Answer from the drawing. Dimensions are ordinates in mm from the lowest x, y and z of the part. A direction names the side the tool comes from. Coordinates: 2 decimals unless noted, no trailing zeros. Write each loop counter-clockwise with the first axis right and the second up, starting at its lowest first coordinate (ties: lowest second). Pieces come first, ordered by that corner, then holes. Notation, with made-up numbers: (89.25, 72.5) - (123.25, 72.5) arc R22 cw to (123.25, 94.5) - close; hole circle Ø4 at (14, -8.5). An arc over 180 degrees is marked (long way). Return JSON: item names as keys, results as strings.
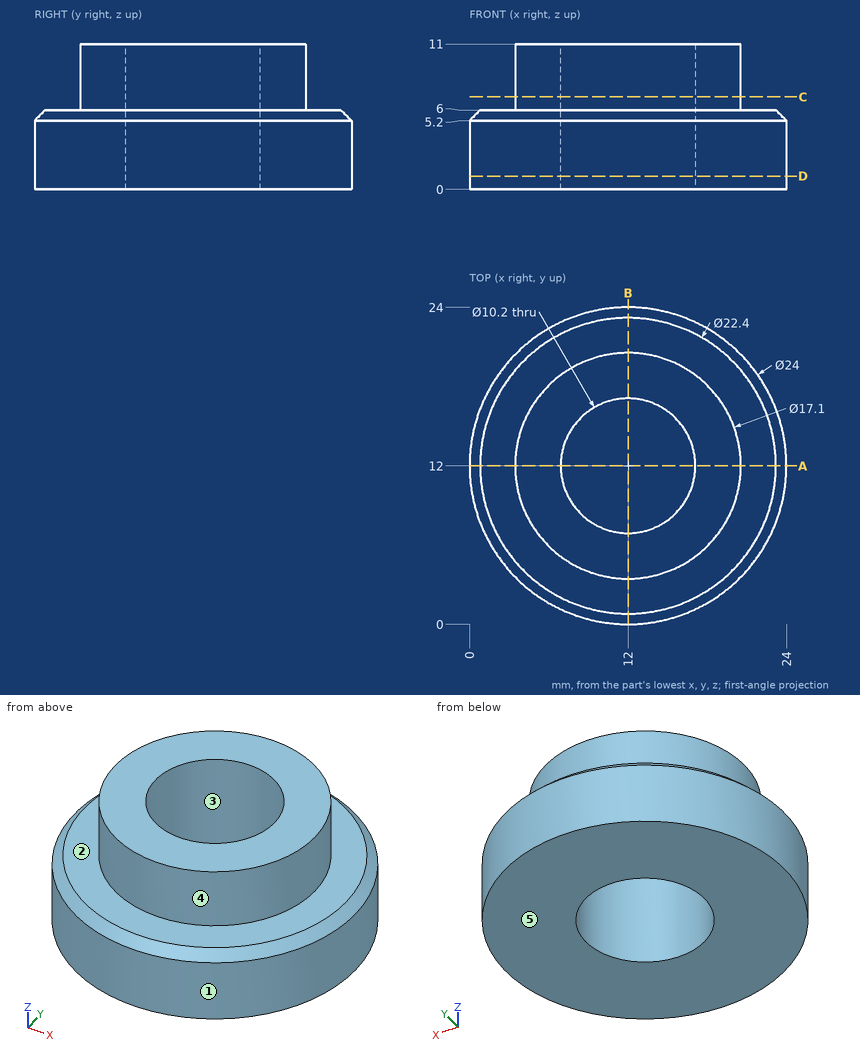
(1) Which of the six approach directions +Z, -Z, +X, -X, +Y, -Y give full straight-line access (tool end or side, diameter ignored) to the marked faces 4 and 5?
Answer:
{"face 4": "+Z", "face 5": "-Z, +X, -X, +Y, -Y"}
(2) Straight lines are drawn through the part: line 1 (Y direction, x = 12, z = 6.5); line 2 (Y direction, x = 12, z = 4.25); line 3 (Z direction, x = 7.25, y = 20.5). For each, find the intervals that lie inside material, in ascending order. Write a range as from..to.
Answer:
{"line 1": "3.45..6.9, 17.1..20.55", "line 2": "0..6.9, 17.1..24", "line 3": "0..6"}
(3) A cutting plane is placed at C-C (z = 7). Determine the outline of the cut face in (x, y), and give its area (3 significant figures).
Answer:
{"outline": "circle Ø17.1 at (12, 12); hole circle Ø10.2 at (12, 12)", "area": "148 mm²"}
(4) A cutting plane is placed at D-D (z = 1). Determine the outline of the cut face in (x, y).
Answer:
{"outline": "circle Ø24 at (12, 12); hole circle Ø10.2 at (12, 12)"}
(5) Flat-ended cylindrical pins translate along their axes: P1, Ø6, axis at x = 12, y = 12, coming from the +Z side (3 decimals); P2, Ø5, axis at y = 17, z = 9, coming from the +X side; P3, Ø5, axis at y = 9.5, z = 6.5, coming from the +X side. Find the tip coordinate at first contact, or state that the pin passes through.
Answer:
{"P1": "through", "P2": "x = 20.18", "P3": "x = 23.99"}
(6) Determine the mould class of the marked faces 1, 2 and 3 for opening direction Y: +Y half, -Y half, draft (parallel to the pull), parting line (faces both ways), or undercut.
Answer:
{"face 1": "parting line", "face 2": "draft", "face 3": "undercut"}
(7) A cutting plane is placed at A-A (y = 12). Determine the outline of the cut face in (x, z).
Answer:
{"outline": "(0, 0) - (6.9, 0) - (6.9, 11) - (3.45, 11) - (3.45, 6) - (0.8, 6) - (0, 5.2) - close; (17.1, 0) - (24, 0) - (24, 5.2) - (23.2, 6) - (20.55, 6) - (20.55, 11) - (17.1, 11) - close"}
